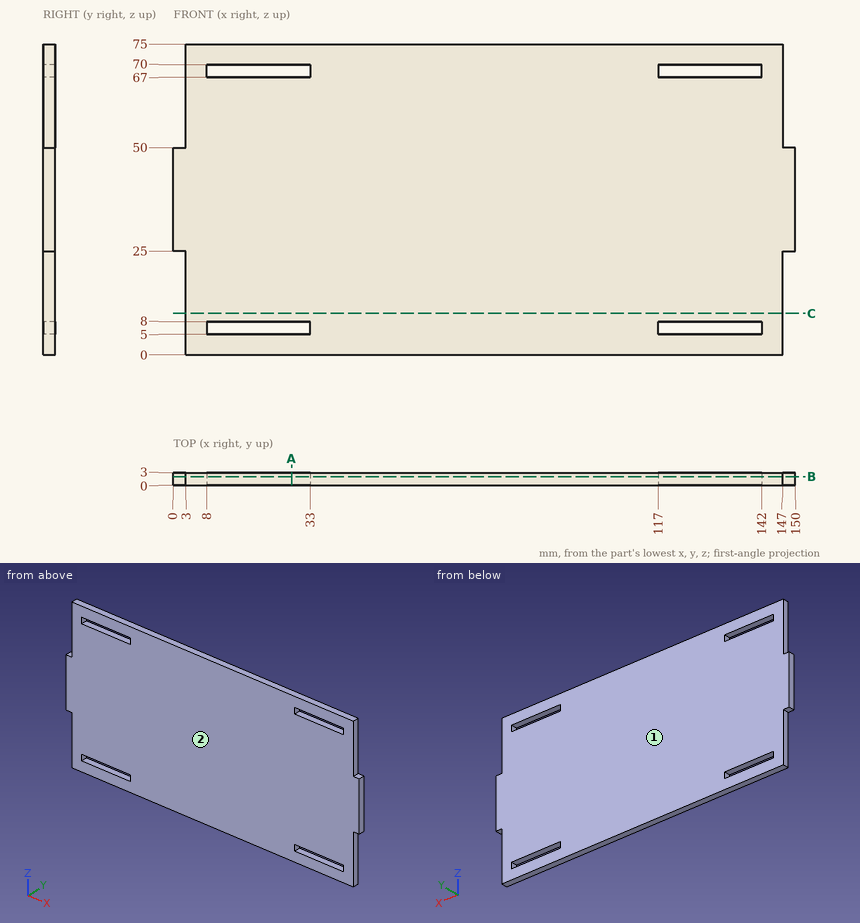
Verification items for this drawing (mm, ordinates from the low corner). Coordinates: 2 decimals unless noted, no trailing zeros. Write each loop counter-clockwise with the first axis right and the second up, starting at its lowest first coordinate (ties: lowest second). Pieces come first, ordered by that corner, then holes. Notation, with made-up numbers: M -28.75,31 L 15.25,31 A20 ccw 15.25,67 Z; hole C 82,74.25 d11. An arc over 180 degrees is marked long. Answer as CSV lines item,"result".
Q1. Material ranges on probe 1 along Z at (x, y) = (120.5, 1); probe 2 along X at (y, z) = (1.85, 6); probe 3 along X at (y, z) = (1.15, 18), recorded low to high. Write a range as from..to.
Check result:
probe 1,"0..5, 8..67, 70..75"
probe 2,"3..8, 33..117, 142..147"
probe 3,"3..147"
Q2. Mould release check, pull along Y, two halves, no side actions. Record for the marked faces 1 and 2: released by +Y, released by -Y, zero draft, split by the parting line, or undercut.
Check result:
face 1,"released by +Y"
face 2,"released by -Y"
Q3. Cross-section at B-B (y = 2.1). Record the boundary of the cut face in (x, z), then the cut area to 4 significant figures.
Check result:
outline,"M 0,25 L 3,25 L 3,0 L 147,0 L 147,25 L 150,25 L 150,50 L 147,50 L 147,75 L 3,75 L 3,50 L 0,50 Z; hole M 8,5 L 33,5 L 33,8 L 8,8 Z; hole M 8,67 L 33,67 L 33,70 L 8,70 Z; hole M 117,5 L 142,5 L 142,8 L 117,8 Z; hole M 117,67 L 142,67 L 142,70 L 117,70 Z"
area,"10,650 mm^2"
Q4. Cross-section at A-A (x = 28.5). Record the boundary of the cut face in (y, z).
Check result:
outline,"M 0,0 L 3,0 L 3,5 L 0,5 Z; M 0,8 L 3,8 L 3,67 L 0,67 Z; M 0,70 L 3,70 L 3,75 L 0,75 Z"
Q5. Cross-section at C-C (z = 10). Record the boundary of the cut face in (x, y), then the cut area to 3 significant figures.
Check result:
outline,"M 3,0 L 147,0 L 147,3 L 3,3 Z"
area,"432 mm^2"
Q6. Go/stop test with flat-tipped pins: pin 1 (0.9 mm diameter, centred on x = 1, y = 1.5, fed in from -Z); pin 2 (0.9 mm diameter, centred on y = 2, z = 6, fed in from -X); pin 3 (0.9 mm diameter, centred on y = 2, z = 6, fed in from +X); pin 4 (1.5 mm diameter, centred on x = 134, y = 1.5, fed in from -Z). Record where each tip stops, or that it passes through.
Check result:
pin 1,"z = 25"
pin 2,"x = 3"
pin 3,"x = 147"
pin 4,"z = 0"
